```python
from build123d import *

# Parameters (mm, degrees)
F0_W      = 127
F0_H      = 50.800004
F1_DEPTH  = 6.35
F2_R      = 4.7625
F2_W      = 9.525
F2_H      = 9.525
F3_DEPTH  = 19.05
F3_FACE_W = 9.525
F3_FACE_H = 9.525
F4_DEPTH  = 6.35


with BuildPart() as f1:
    # F0 (on Right) → F1 (new body)
    with BuildSketch(Plane.YZ):
        Rectangle(F0_W, F0_H)
    extrude(amount=F1_DEPTH)

    # F2 (on face) → F3 (join)
    with BuildSketch(Plane.YZ.offset(6.35)):
        with Locations((-38.1, 0)):
            Circle(F2_R)
        with Locations((38.1, 0)):
            Rectangle(F2_W, F2_H)
    extrude(amount=F3_DEPTH)

    # F3_face (on face) → F4 (join)
    with BuildSketch(Plane(origin=(25.4, 38.1, 0), x_dir=(0, 1, 0), z_dir=(1, 0, 0))):
        Rectangle(F3_FACE_W, F3_FACE_H)
    extrude(amount=F4_DEPTH)


solid = f1.part
```
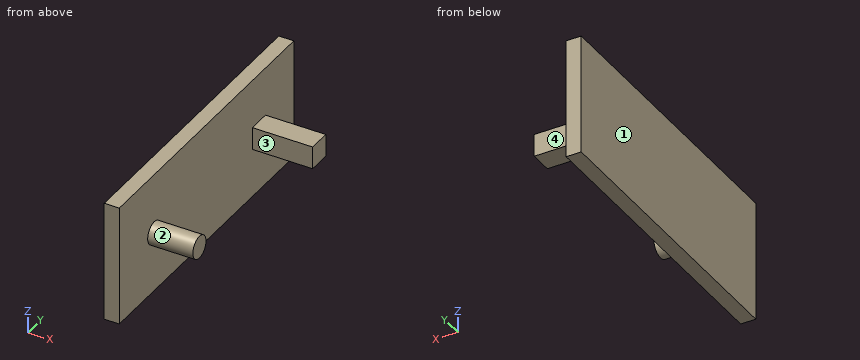
Model file for the job. Use its own axes, mm. Face numbers are marked on the shaded views. A direction names the side the tool comes from. Give positions to 0.01 mm unless a question says otherwise; leave off trailing zeros. Write each loop counter-clockwise with the first axis right and the second up, starting at its lowest first coordinate (ties: lowest second). Pieces come first, ordered by that corner, then holes. Notation, with made-up numbers: M 45,11 L 97,11 A11 ccw 97,31 Z; hole C 32.5,12 d6. An arc over 180 degrees is marked long. Use a Markdown table: item, result.
1) Drill centre lines: line 1 (X direction, y = 13, z = 6); line 2 (Z direction, x = 21.5, y = -34); line 3 (Z direction, x = 19, y = -41). Where is each one in solid material? Low to high. Write a range as from..to.
Responses:
| item | result |
|---|---|
| line 1 | x = 0..6.35 |
| line 2 | z = -2.42..2.42 |
| line 3 | z = -3.78..3.78 |
2) Cut at B-B (y = -38.1). List the corners of the cut face in (x, z).
Responses:
| item | result |
|---|---|
| outline | M 0,-25.4 L 6.35,-25.4 L 6.35,-4.76 L 25.4,-4.76 L 25.4,4.76 L 6.35,4.76 L 6.35,25.4 L 0,25.4 Z |
3) Tool access for the marked faces 1, 2, 3 and 4: list every direction of +Z, -Z, +X, -X, +Y, -Y with a clear straight run to the whole face (end or side of a thin tool).
Responses:
| item | result |
|---|---|
| face 1 | +Z, -Z, -X, +Y, -Y |
| face 2 | +X |
| face 3 | +Z, -Z, +X |
| face 4 | +Z, -Z, +X, +Y |
4) Cut at A-A (z = 0). List the corners of the cut face in (x, y).
Responses:
| item | result |
|---|---|
| outline | M 0,-63.5 L 6.35,-63.5 L 6.35,-42.86 L 25.4,-42.86 L 25.4,-33.34 L 6.35,-33.34 L 6.35,33.34 L 31.75,33.34 L 31.75,42.86 L 6.35,42.86 L 6.35,63.5 L 0,63.5 Z |
5) Cut at D-D (z = -7). List the corners of the cut face in (x, y), and give its area (3 significant figures).
Responses:
| item | result |
|---|---|
| outline | M 0,-63.5 L 6.35,-63.5 L 6.35,63.5 L 0,63.5 Z |
| area | 806 mm2 |
6) Cut at C-C (y = 25). List the corners of the cut face in (x, z).
Responses:
| item | result |
|---|---|
| outline | M 0,-25.4 L 6.35,-25.4 L 6.35,25.4 L 0,25.4 Z |
7) Pin check, flat tips, straight feed: pin 1 (4 mm diameter, centred on y = -9, z = -19.5, fed in from +X); pin 2 (5 mm diameter, centred on x = 13.5, y = 38, fed in from +Z); pin 3 (10.5 mm diameter, centred on x = 23.5, z = 2, fed in from -Y). Stop position of each tip, or through.
Responses:
| item | result |
|---|---|
| pin 1 | stops at x = 6.35 |
| pin 2 | stops at z = 4.76 |
| pin 3 | stops at y = -42.86 |
